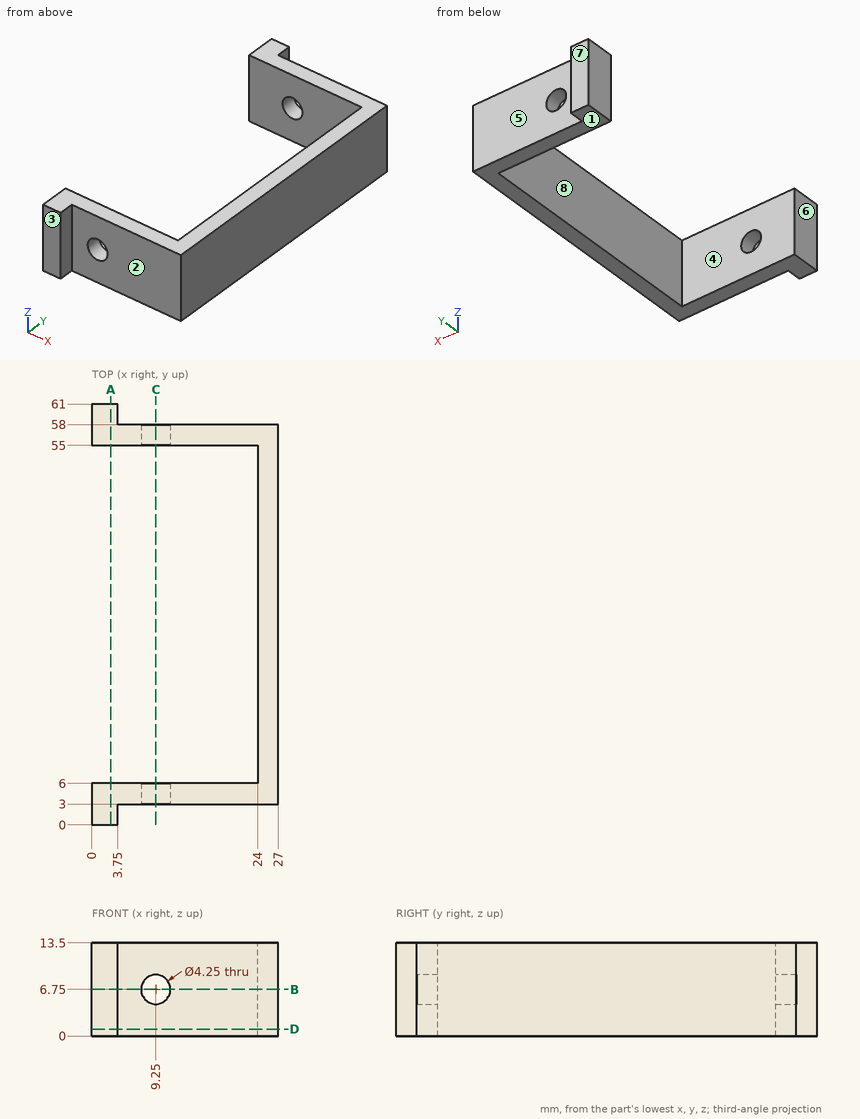
The drawing under review shows one solid part. Ordinate dimensions are in mm from its lowest x, y, z. A direction names the side the tool comes from. Round coordinates to 2 decimals unless told otherwise and drop trailing zeros. Order: outer loops, then holes, each group sorted by start corner. A loop starts at its lowest first (then second) coordinate and runs counter-clockwise, first axis right, second up. Notation, with made-up numbers: (10.5, -36.75) - (47.5, -36.75) arc R25 ccw to (47.5, -11.75) - close; hole circle Ø8 at (87.5, 86). An arc over 180 degrees is marked (long way). Return JSON: item names as keys, results as strings.
Q1. For pin 1 Ø1 at (y, z) = (20.5, 4.5) entering from -X; pin 2 Ø7 at (x, z) = (13, 8.5) entering from +Y; pin 3 Ø7 at (x, z) = (15, 7) entering from -Y; pin 4 Ø10 at (x, y) = (7, 49) entering from -Z (1 decimal), all flat-tipped, find the tip position at first contact; note any pin that passes through.
Computed values:
{"pin 1": "stops at x = 24", "pin 2": "stops at y = 58", "pin 3": "stops at y = 3", "pin 4": "passes through"}
Q2. The part is to be moulded in two halves that separate along Y. For the marked faces 6, 7 and 8, say which applies: pulls with the +Y half, pulls with the -Y half, needs draft (parallel to the pull), parting line crosses it, or undercut.
Computed values:
{"face 6": "needs draft", "face 7": "pulls with the +Y half", "face 8": "undercut"}
Q3. Machinability: for the marked faces 1, 2, 3, 4 and 5, which of the approach directions +Z, -Z, +X, -X, +Y, -Y give a long, thin tool a straight path to every point of the face, cutting with its end or side? Answer none if there is none.
Computed values:
{"face 1": "-Z, +X, -X, +Y, -Y", "face 2": "+Z, -Z, +X, -Y", "face 3": "+Z, -Z, +X, -X, -Y", "face 4": "+Z, -Z, -X", "face 5": "+Z, -Z, +X, +Y"}
Q4. Consider section B-B on z = 6.75. Write out the cut boundary in (x, y) (3 decimals), plus the area to 3 significant figures.
Computed values:
{"outline": "(0, 0) - (3.75, 0) - (3.75, 3) - (7.125, 3) - (7.125, 6) - (0, 6) - close; (0, 55) - (7.125, 55) - (7.125, 58) - (3.75, 58) - (3.75, 61) - (0, 61) - close; (11.375, 3) - (27, 3) - (27, 58) - (11.375, 58) - (11.375, 55) - (24, 55) - (24, 6) - (11.375, 6) - close", "area": "306 mm2"}
Q5. Consider section D-D on z = 1. Write out the cut boundary in (x, y).
Computed values:
{"outline": "(0, 0) - (3.75, 0) - (3.75, 3) - (27, 3) - (27, 58) - (3.75, 58) - (3.75, 61) - (0, 61) - (0, 55) - (24, 55) - (24, 6) - (0, 6) - close"}
Q6. Consider section C-C on x = 9.25. Write out the cut boundary in (y, z) (3 decimals), plus the area to 3 significant figures.
Computed values:
{"outline": "(3, 0) - (6, 0) - (6, 4.625) - (3, 4.625) - close; (3, 8.875) - (6, 8.875) - (6, 13.5) - (3, 13.5) - close; (55, 0) - (58, 0) - (58, 4.625) - (55, 4.625) - close; (55, 8.875) - (58, 8.875) - (58, 13.5) - (55, 13.5) - close", "area": "55.5 mm2"}
Q7. Consider section A-A on x = 2.75. Write out the cut boundary in (y, z), plus the area to 3 significant figures.
Computed values:
{"outline": "(0, 0) - (6, 0) - (6, 13.5) - (0, 13.5) - close; (55, 0) - (61, 0) - (61, 13.5) - (55, 13.5) - close", "area": "162 mm2"}
Q8. Wall thickness on L1, parallel to Y at x = 19, z = 1.5; L2, parallel to X at y = 5.35, z = 6.75 (3 decimals); L3, parallel to Y at x = 2.75, z = 4.25: over which ranges is each line inside the solid? List them lowest first. Write a range as [from, to].
Computed values:
{"L1": "y = [3, 6], [55, 58]", "L2": "x = [0, 7.125], [11.375, 27]", "L3": "y = [0, 6], [55, 61]"}
